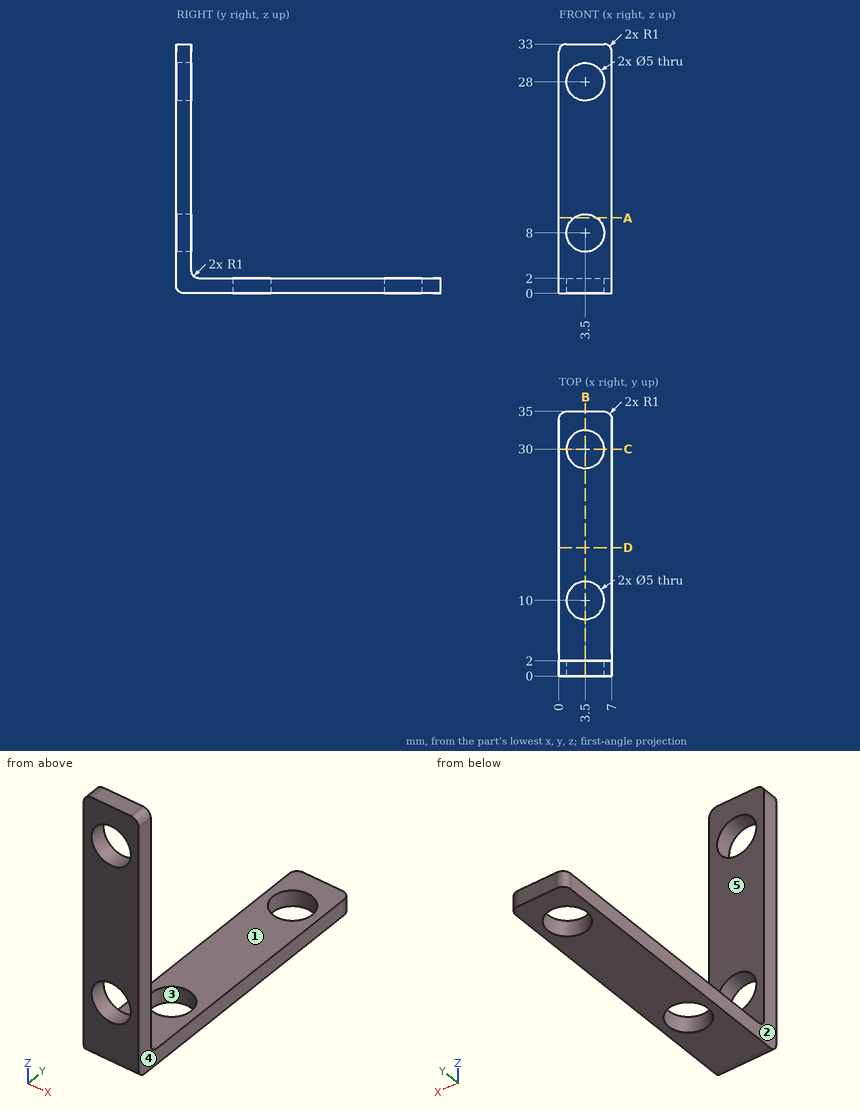
Design review of the part shown in the three views and the two pictorial views. Dimensions are in mm from the part's minimum x, y and z. A direction names the side the tool comes from. Coordinates: 2 decimals unless noted, no trailing zeros. Loops run counter-clockwise (first coordinate to the right, second up) from the corner with the lowest first, then second, coordinate; pieces in that order, holes last.
Q1. Tool access review of the marked faces 1 and 2: name each direction out of +Z, -Z, +X, -X, +Y, -Y from which nothing blocks a thin tool from reaching the whole face with its end or side.
Reported:
face 1: +Z, +X, -X, +Y
face 2: +Z, -Z, -X, +Y, -Y
Q2. We need section C-C on y = 30. State the section outline as (x, z) points.
Reported:
outline: (0, 0) - (1, 0) - (1, 2) - (0, 2) - close; (6, 0) - (7, 0) - (7, 2) - (6, 2) - close
Q3. To check wall thickness, follow line 1 (Y direction, x = 3.5, z = 1.25); line 2 (Z direction, x = 4, y = 17). State the ranges of each line that lie inside material, in increasing order.
Reported:
line 1: y = 0 to 7.5, 12.5 to 27.5, 32.5 to 35
line 2: z = 0 to 2
Q4. The part is to be moulded in two halves that separate along Y. For the marked faces 3, 4 and 5, say which applies: +Y half, -Y half, draft (parallel to the pull), parting line (faces both ways), or undercut.
Reported:
face 3: undercut
face 4: draft
face 5: +Y half
Q5. For pin 1 (4 mm diameter, centred on x = 3.5, z = 28, fed in from -Y); pin 2 (3 mm diameter, centred on x = 5, z = 28, fed in from +Y); pin 3 (3.5 mm diameter, centred on x = 3.5, y = 16.5, fed in from +Z), all flat-tipped, find the tip position at first contact; note any pin that passes through.
Reported:
pin 1: passes through
pin 2: stops at y = 2
pin 3: stops at z = 2
Q6. We need section D-D on y = 17. State the section outline as (x, z) points, and give its area (3 significant figures).
Reported:
outline: (0, 0) - (7, 0) - (7, 2) - (0, 2) - close
area: 14.0 mm2
Q7. We need section B-B on x = 3.5. State the section outline as (y, z) points, and give its area (3 significant figures).
Reported:
outline: (0, 1) arc R1 ccw to (1, 0) - (7.5, 0) - (7.5, 2) - (3, 2) arc R1 cw to (2, 3) - (2, 5.5) - (0, 5.5) - close; (0, 10.5) - (2, 10.5) - (2, 25.5) - (0, 25.5) - close; (0, 30.5) - (2, 30.5) - (2, 33) - (0, 33) - close; (12.5, 0) - (27.5, 0) - (27.5, 2) - (12.5, 2) - close; (32.5, 0) - (35, 0) - (35, 2) - (32.5, 2) - close
area: 92.0 mm2
Q8. We need section A-A on z = 10. State the section outline as (x, y) points, and give its area (3 significant figures).
Reported:
outline: (0, 0) - (2, 0) - (2, 2) - (0, 2) - close; (5, 0) - (7, 0) - (7, 2) - (5, 2) - close
area: 8.00 mm2
